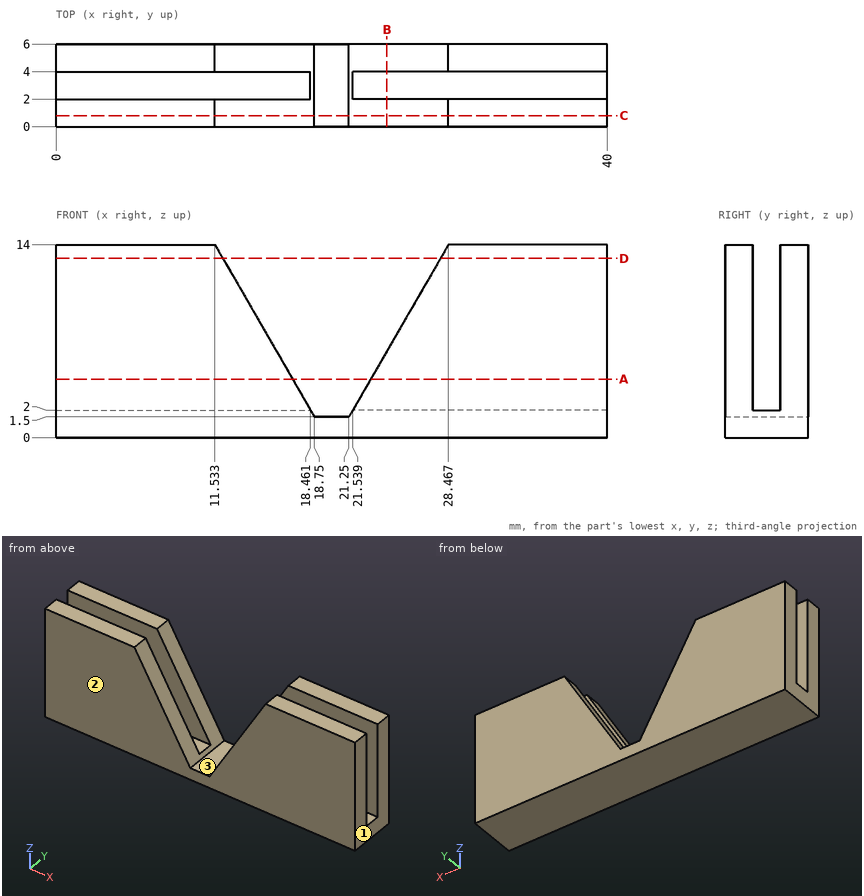
Verification items for this drawing (mm, ordinates from the low corner). Give positions to 0.01 mm unless a question says otherwise; leave off trailing zeros. Loops run counter-clockwise (first coordinate to the right, second up) from the corner with the lowest first, then second, coordinate; pieces in that order, holes last. Notation, with made-up numbers: (-2.75, -0.5) - (31.25, -0.5) arc R18 cw to (31.25, 25.5) - close; hole circle Ø10 at (53, 45). An arc over 180 degrees is marked (long way). Write item = value, one per line. Start each with the question number.
Q1. Thickness scan on line 1 (Y direction, x = 12.5, z = 11.25); line 2 (Z direction, x = 36.5, y = 3.7); line 3 (X direction, y = 5.4, z = 11.25). Record the ranges inside material, lowest first.
Q2. Mould release check, pull along X, two halves, no side actions. Record for the marked faces 1, 2 and 3: released by +X, released by -X, zero draft, split by the parting line, or undercut.
Q3. Cross-section at D-D, the plane z = 13. Enter the section's corners in (x, y).
Q4. Cross-section at C-C, the plane y = 0.8. Enter the section's corners in (x, z).
Q5. Cross-section at B-B, the plane x = 24. Enter the section's corners in (y, z).
Q6. Depth check by flat-ended pin: P1, Ø0.8, axis at x = 19.5, y = 4, coming from the +Z side. Enter the tip coordinate at first touch or a pass-through.
Q7. Cross-section at A-A, the plane z = 4.25. Enter the section's corners in (x, y), and give its area (3 significant figures).
Answer key:
q1.line_1 = 0 to 2, 4 to 6
q1.line_2 = 0 to 2
q1.line_3 = 0 to 13.12, 26.88 to 40
q2.face_1 = released by +X
q2.face_2 = zero draft
q2.face_3 = undercut
q3.outline = (0, 0) - (12.11, 0) - (12.11, 2) - (0, 2) - close; (0, 4) - (12.11, 4) - (12.11, 6) - (0, 6) - close; (27.89, 0) - (40, 0) - (40, 2) - (27.89, 2) - close; (27.89, 4) - (40, 4) - (40, 6) - (27.89, 6) - close
q4.outline = (0, 0) - (40, 0) - (40, 14) - (28.47, 14) - (21.25, 1.5) - (18.75, 1.5) - (11.53, 14) - (0, 14) - close
q5.outline = (0, 0) - (6, 0) - (6, 6.26) - (4, 6.26) - (4, 2) - (2, 2) - (2, 6.26) - (0, 6.26) - close
q6.P1 = 1.5
q7.outline = (0, 0) - (17.16, 0) - (17.16, 2) - (0, 2) - close; (0, 4) - (17.16, 4) - (17.16, 6) - (0, 6) - close; (22.84, 0) - (40, 0) - (40, 2) - (22.84, 2) - close; (22.84, 4) - (40, 4) - (40, 6) - (22.84, 6) - close
q7.area = 137 mm^2
